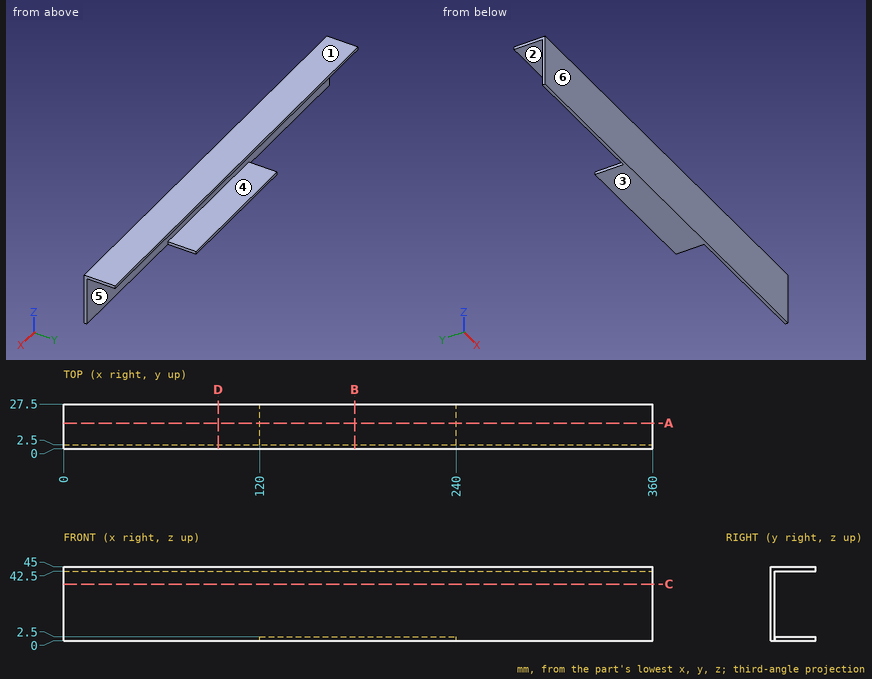
Source: three-view drawing plus pictorial views. Frame: mm from the lowest corner of the part. A direction names the side the tool comes from. Coordinates: 2 decimals unless noted, no trailing zeros. Order: outer loops, then holes, each group sorted by start corner. A loop starts at its lowest first (then second) coordinate and runs counter-clockwise, first axis right, second up.
Item 1: Cut plane A-A (y = 15.75). Return loops of the section in (x, z).
Output values:
outline: (0, 42.5) - (360, 42.5) - (360, 45) - (0, 45) - close; (120, 0) - (240, 0) - (240, 2.5) - (120, 2.5) - close
Item 2: Cut plane B-B (x = 178). Return loops of the section in (y, z), plus the area to 4 significant figures.
Output values:
outline: (0, 0) - (27.5, 0) - (27.5, 2.5) - (2.5, 2.5) - (2.5, 42.5) - (27.5, 42.5) - (27.5, 45) - (0, 45) - close
area: 237.5 mm2
Item 3: Cut plane D-D (x = 94.5). Return loops of the section in (y, z).
Output values:
outline: (0, 0) - (2.5, 0) - (2.5, 42.5) - (27.5, 42.5) - (27.5, 45) - (0, 45) - close
Item 4: Cut plane C-C (z = 34.5). Return loops of the section in (x, y).
Output values:
outline: (0, 0) - (360, 0) - (360, 2.5) - (0, 2.5) - close
Item 5: Material intervals for line 1 (Z direction, x = 150.5, y = 20.5); line 2 (Z direction, x = 301.5, y = 10.25); line 3 (Y direction, x = 112.5, z = 16.5), sorted ascending.
Output values:
line 1: z = 0 to 2.5, 42.5 to 45
line 2: z = 42.5 to 45
line 3: y = 0 to 2.5
Item 6: First-contact query: P1, Ø6, axis at x = 299, y = 22.5, coming from the -Z side; P2, Ø5, axis at x = 210, z = 34.5, coming from the +Y side; P3, Ø2, axis at y = 12, z = 1.5, coming from the +X side. Flat tips, straight axial feed; report the tip coordinate or a pass-through.
Output values:
P1: stops at z = 42.5
P2: stops at y = 2.5
P3: stops at x = 240
Item 7: Set-up query: the marked faces 1 and 2. Return all of +Z, -Z, +X, -X, +Y, -Y with unobstructed straight access to the full face (end or side cutting, diameter ignored); none if empty.
Output values:
face 1: +Z, +X, -X, +Y, -Y
face 2: +X, -X, +Y
Item 8: Pull-direction query (Z, two-part tool) for the marked faces 3, 4, 5 and 6; classes: pulls with the +Z half, pulls with the -Z half, needs draft (parallel to the pull), parting line crosses it, or undercut.
Output values:
face 3: pulls with the -Z half
face 4: undercut
face 5: undercut
face 6: needs draft
